Check sheet for the drawn part. Datum: minimum x, y, z corner. Units: mm. A direction names the side the tool comes from. Give positions to 0.01 mm unless a question says otherwise; leave off trailing zeros. Write each loop counter-clockwise with the first axis right and the second up, starting at its lowest first coordinate (ties: lowest second). Pieces come first, ordered by that corner, then holes. Notation, with made-up numbers: (40, 20) -> (94, 20) arc R14 cw to (94, 35) -> close; hole circle Ø2 at (84, -25.5). An arc over 180 degrees is marked (long way). Answer as CSV lines item,"result". Start each with the question number.
1) Mould release check, pull along X, two halves, no side actions. Record for the marked faces 4, 5, 6 and 7: released by +X, released by -X, zero draft, split by the parting line, or undercut.
2) Gauge pin test, flat ends, axial feed: pin 1 Ø2.5 at (y, z) = (4, 3.5) entering from -X (1 decimal); pin 2 Ø2.5 at (y, z) = (21, 2.5) entering from -X (1 decimal). Record the tip position at first contact, or that the pin passes through.
3) Material ranges on L1, parallel to X at y = 4, z = 3.45 (1 decimal); L2, parallel to Y at x = 9.25, z = 1.6; L3, parallel to Y at x = 17.25, z = 2.85, recorded low to high.
4) Tool access check on the marked faces 1, 2 and 3. Record the directions out of +Z, -Z, +X, -X, +Y, -Y that give a thin tool (end or side, any length) a straight path to the whole face; none if there is none.
5) Sectioned sample at C-C on y = 25. Record the cut outline in (x, z) (1 decimal).
6) Sectioned sample at B-B on x = 5.75. Record the cut outline in (y, z), and give its area (3 significant figures).
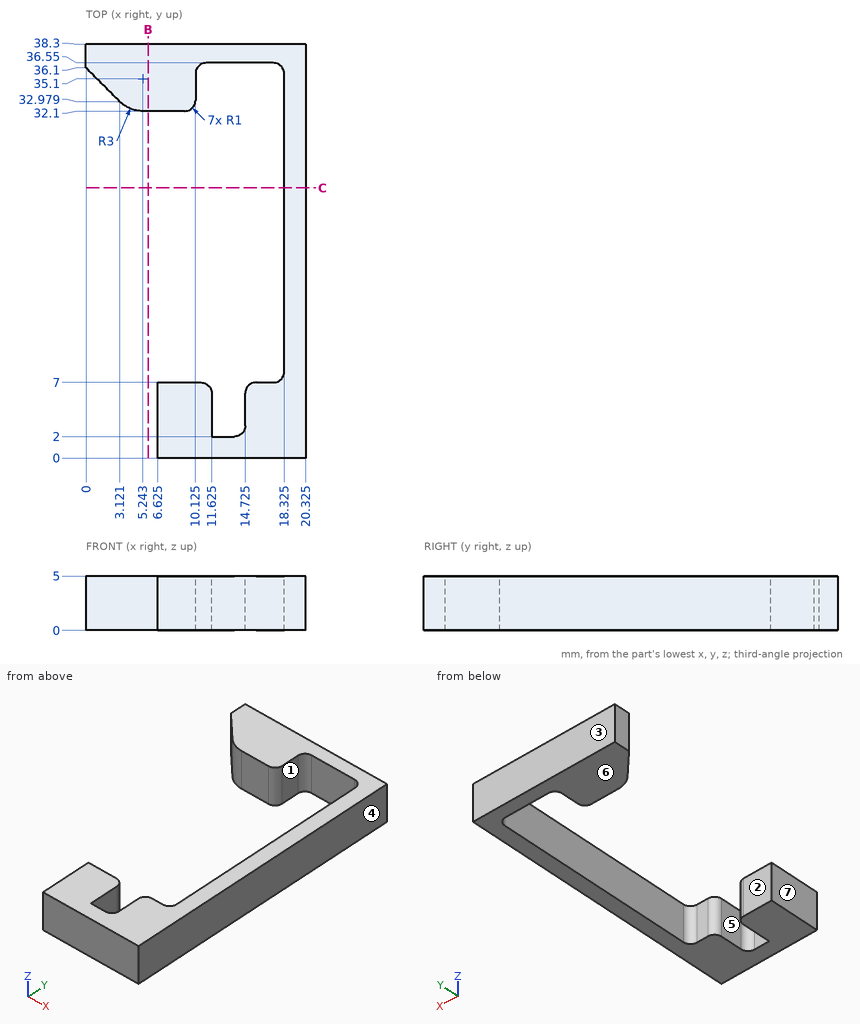
Ans:
1,face 4,"released by +X"
1,face 5,"undercut"
1,face 6,"zero draft"
1,face 7,"released by -X"
2,pin 1,"stops at x = 6.6"
2,pin 2,"stops at x = 18.3"
3,L1,"x = 6.6 to 11.6, 14.7 to 20.3"
3,L2,"y = 0 to 7, 32.11 to 38.3"
3,L3,"y = 0 to 7, 36.55 to 38.3"
4,face 1,"+Z, -Z"
4,face 2,"+Z, -Z, -X"
4,face 3,"+Z, -Z, +X, -X, +Y"
5,outline,"(18.3, 0) -> (20.3, 0) -> (20.3, 5) -> (18.3, 5) -> close"
6,outline,"(32.1, 0) -> (38.3, 0) -> (38.3, 5) -> (32.1, 5) -> close"
6,area,"31.0 mm²"
